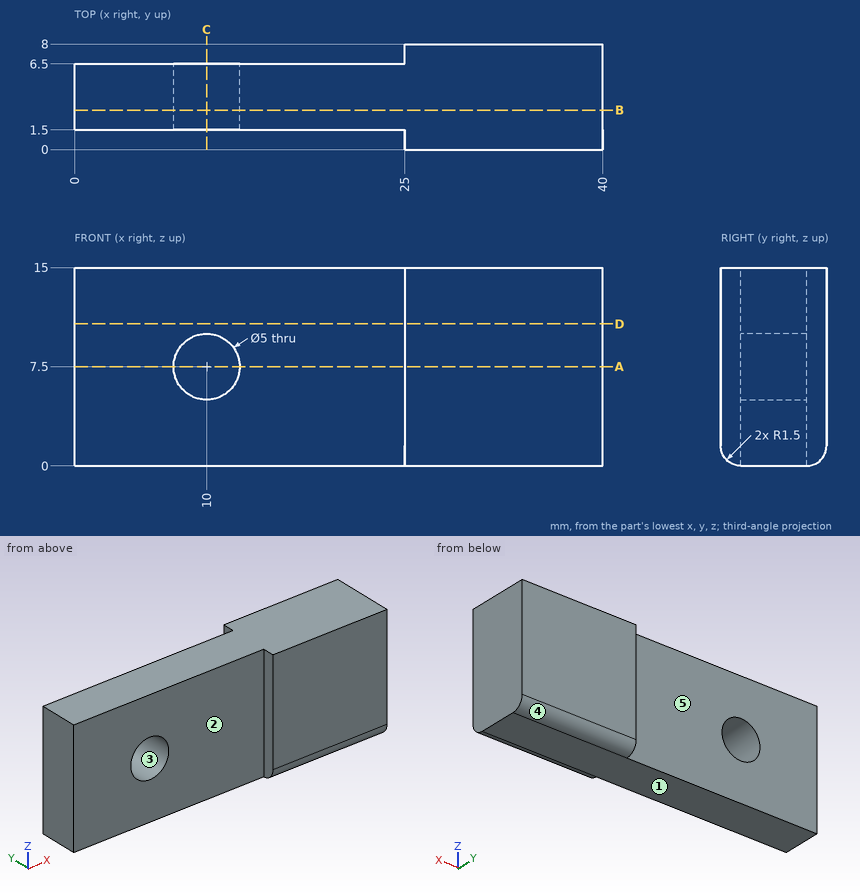
Verification items for this drawing (mm, ordinates from the low corner). A direction names the side the tool comes from. Give positions to 0.01 mm unless a question says otherwise; leave off trailing zeros. Loops run counter-clockwise (first coordinate to the right, second up) from the corner with the lowest first, then second, coordinate; pieces in that order, holes last. Notation, with made-up numbers: (-31.75, -11.5) - (-6.75, -11.5) arc R21 cw to (-6.75, 27.5) - close; hole circle Ø6 at (61, -0.75). An arc over 180 degrees is marked (long way). Write item = value, one per line. Start each with the question number.
Q1. Thickness scan on line 1 (X direction, y = 2.9, z = 7.5); line 2 (X direction, y = 1.25, z = 5.5); line 3 (Y direction, x = 24, z = 12.25). Record the ranges inside material, lowest first.
Q2. Tool access check on the marked faces 1 and 2. Record the directions out of +Z, -Z, +X, -X, +Y, -Y that give a thin tool (end or side, any length) a straight path to the whole face; none if there is none.
Q3. Cross-section at B-B, the plane y = 3. Enter the section's corners in (x, z), and give its area (3 significant figures).
Q4. Cross-section at A-A, the plane z = 7.5. Enter the section's corners in (x, y), and give its area (3 significant figures).
Q5. Mould release check, pull along Z, two halves, no side actions. Record for the marked faces 3, 4 and 5: released by +Z, released by -Z, zero draft, split by the parting line, or undercut.
Q6. Depth check by flat-ended pin: P1, Ø1.2, axis at y = 7.5, z = 11, coming from the -X side; P2, Ø4.5, axis at x = 10, z = 7.5, coming from the -Y side; P3, Ø8, axis at x = 10, z = 4.5, coming from the -Y side; P4, Ø2, axis at x = 18.5, z = 4, coming from the +Y side. Enter the tip coordinate at first touch or a pass-through.
Q7. Cross-section at D-D, the plane z = 10.75. Enter the section's corners in (x, y).
Q8. Cross-section at C-C, the plane x = 10. Enter the section's corners in (y, z).
Answer key:
q1.line_1 = 0 to 7.5, 12.5 to 40
q1.line_2 = 25 to 40
q1.line_3 = 1.5 to 6.5
q2.face_1 = -Z, +X, -X, +Y, -Y
q2.face_2 = +Z, -Z, -X, -Y
q3.outline = (0, 0) - (40, 0) - (40, 15) - (0, 15) - close; hole circle Ø5 at (10, 7.5)
q3.area = 580 mm^2
q4.outline = (0, 1.5) - (7.5, 1.5) - (7.5, 6.5) - (0, 6.5) - close; (12.5, 1.5) - (25, 1.5) - (25, 0) - (40, 0) - (40, 8) - (25, 8) - (25, 6.5) - (12.5, 6.5) - close
q4.area = 220 mm^2
q5.face_3 = undercut
q5.face_4 = released by -Z
q5.face_5 = zero draft
q6.P1 = 25
q6.P2 = through
q6.P3 = 1.5
q6.P4 = 6.5
q7.outline = (0, 1.5) - (25, 1.5) - (25, 0) - (40, 0) - (40, 8) - (25, 8) - (25, 6.5) - (0, 6.5) - close
q8.outline = (1.5, 0) - (6.5, 0) - (6.5, 5) - (1.5, 5) - close; (1.5, 10) - (6.5, 10) - (6.5, 15) - (1.5, 15) - close
